Geometry check sheet. Reference: the model listing, model coordinates, mm. A direction names the side the tool comes from. Coordinates: 2 decimals unless noted, no trailing zeros. Write each loop counter-clockwise with the first axis right and the second up, starting at its lowest first coordinate (ties: lowest second). Pieces come first, ordered by that corner, then holes. Notation, with made-up numbers: (54, 22) -> (74, 22) arc R9 ccw to (74, 36) -> close; hole circle Ø3 at (7, 46.25). An arc over 180 degrees is marked (long way). Answer in a Markdown table with one row per item. Add a question column.
Q1. Release check for a two-part mould opening along X. For faces 1 (the face through (14.628, 70, 7)), 2 (the face through (9.628, 81, 7)), 3 (the face through (-77.372, -16, 7)), 4 (the face through (12, 95.77, 7)) record: pulls with the +X half, pulls with the -X half, needs draft (parallel to the pull), parting line crosses it, or undercut.
Q2. Section check C-C, the plane x = -27.5. Record the boundary of the cut face in (y, z).
Q3. Tool access check on faces 5 (the face through (-29, 29, 15)), 6 (the face through (-18.872, 17, 7)), 7 (the face through (-28, 55.77, 7)), 8 (the face through (-56, 45.77, 7)), 9 (the face through (-72.372, 71, 7)). Record the directions out of +Z, -Z, +X, -X, +Y, -Y that give a thin tool (end or side, any length) a straight path to the whole face; none if there is none.
Q4. Section check B-B, the plane z = 13.75. Record the boundary of the cut face in (x, y), and give its area (3 significant figures).
Q5. Section check A-A, the plane x = -45.5. Record the boundary of the cut face in (y, z), and give its area (3 significant figures).
Q6. Section check D-D, the plane y = 11.5. Record the boundary of the cut face in (x, z).
Q7. Thickness scan on line 1 (Y direction, x = -50.5, z = 10.5); line 2 (X direction, y = 76, z = 8); line 3 (Y direction, x = -71, z = 3.5). Record the ranges inside material, lowest first.
Q8. Gauge pin test, flat ends, axial feed: P1, Ø7.5, axis at y = 22, z = 6, coming from the -X side; P2, Ø4.5, axis at y = 61, z = 5, coming from the -X side; P3, Ø8, axis at x = -56, z = 6, coming from the +Y side; P4, Ø6, axis at x = -37.5, y = 10.5, coming from the -Z side. Record the tip position at first contact, or that the pin passes through.
```python
from build123d import *

# Parameters (mm, degrees)
SKETCH_1_W      = 5
SKETCH_1_H      = 40
SKETCH_1_W_2    = 20
SKETCH_1_H_2    = 57
SKETCH_1_W_3    = 97
SKETCH_1_H_3    = 10
EXTRUDE_1_DEPTH = 15
FILLET_1_R      = 10


with BuildPart() as part:
    # 草圖1 → 填料-伸長1 (new body)
    with BuildSketch(Plane.XY):
        with Locations((-69.872316496, 75.770491803)):
            Rectangle(SKETCH_1_W, SKETCH_1_H)
        Polygon((-72.372316496, 45.770491803), (-38.872316496, 45.770491803), (-18.872316496, 45.770491803), (14.627683504, 45.770491803), (14.627683504, 55.770491803), (9.627683504, 55.770491803), (-67.372316496, 55.770491803), (-72.372316496, 55.770491803), align=None)
        with Locations((12.127683504, 75.770491803)):
            Rectangle(SKETCH_1_W, SKETCH_1_H)
        with Locations((-28.872316496, 17.270491803)):
            Rectangle(SKETCH_1_W_2, SKETCH_1_H_2)
        with Locations((-28.872316496, -16.229508197)):
            Rectangle(SKETCH_1_W_3, SKETCH_1_H_3)
    extrude(amount=EXTRUDE_1_DEPTH)

    # 圓角1
    fillet_1_edges = [part.edges().sort_by_distance(p)[0] for p in [
        (-67.372316496, 55.770491803, 7.5),
        (9.627683504, 55.770491803, 7.5),
    ]]
    fillet(fillet_1_edges, radius=FILLET_1_R)


solid = part.part
```
Calculated:
| question | item | result |
|---|---|---|
| 1 | face 1 | pulls with the +X half |
| 1 | face 2 | undercut |
| 1 | face 3 | pulls with the -X half |
| 1 | face 4 | needs draft |
| 2 | outline | (-21.23, 0) -> (55.77, 0) -> (55.77, 15) -> (-21.23, 15) -> close |
| 3 | face 5 | +Z, +X, -X, +Y, -Y |
| 3 | face 6 | +Z, -Z, +X |
| 3 | face 7 | +Z, -Z, +Y |
| 3 | face 8 | +Z, -Z, -X |
| 3 | face 9 | +Z, -Z, -X, +Y |
| 4 | outline | (-77.37, -21.23) -> (19.63, -21.23) -> (19.63, -11.23) -> (-18.87, -11.23) -> (-18.87, 45.77) -> (14.63, 45.77) -> (14.63, 95.77) -> (9.63, 95.77) -> (9.63, 65.77) arc R10 cw to (-0.37, 55.77) -> (-57.37, 55.77) arc R10 cw to (-67.37, 65.77) -> (-67.37, 95.77) -> (-72.37, 95.77) -> (-72.37, 45.77) -> (-38.87, 45.77) -> (-38.87, -11.23) -> (-77.37, -11.23) -> close |
| 4 | area | 3,420 mm² |
| 5 | outline | (-21.23, 0) -> (-11.23, 0) -> (-11.23, 15) -> (-21.23, 15) -> close; (45.77, 0) -> (55.77, 0) -> (55.77, 15) -> (45.77, 15) -> close |
| 5 | area | 300 mm² |
| 6 | outline | (-38.87, 0) -> (-18.87, 0) -> (-18.87, 15) -> (-38.87, 15) -> close |
| 7 | line 1 | y = -21.23 to -11.23, 45.77 to 55.77 |
| 7 | line 2 | x = -72.37 to -67.37, 9.63 to 14.63 |
| 7 | line 3 | y = -21.23 to -11.23, 45.77 to 95.77 |
| 8 | P1 | stops at x = -38.87 |
| 8 | P2 | stops at x = -72.37 |
| 8 | P3 | stops at y = 56.12 |
| 8 | P4 | stops at z = 0 |
